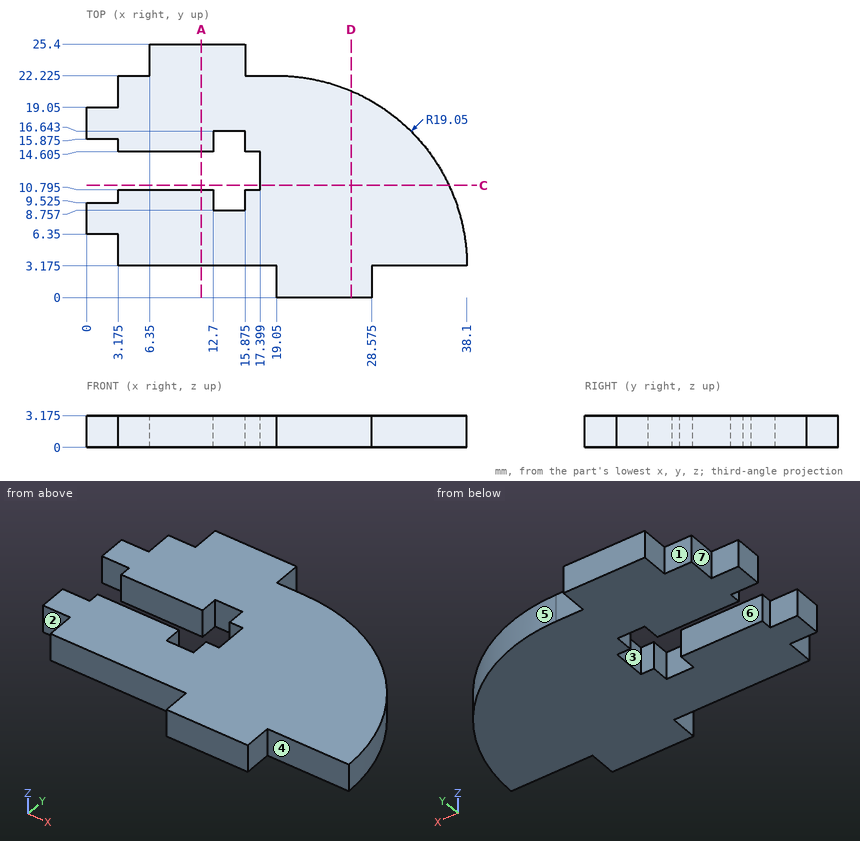
Geometry: see drawing. Coordinates: mm, zero at the bounding-box minimum. A direction names the side the tool comes from. Coordinates: 2 decimals unless noted, no trailing zeros. Loops run counter-clockwise (first coordinate to the right, second up) from the corner with the lowest first, then second, coordinate; pieces in that order, holes last. Notation, with made-up numbers: M 66.5,21.25 L 86.5,21.25 A13 cw 86.5,26.25 Z; hole C 46.5,88.25 d1. An arc over 180 degrees is marked long. Answer in a Markdown table with one row per item.
Q1. Section A-A on x = 11.5. Return the cut outline in (y, z) (1 decimal).
Answers below:
| item | result |
|---|---|
| outline | M 3.2,0 L 10.8,0 L 10.8,3.2 L 3.2,3.2 Z; M 14.6,0 L 25.4,0 L 25.4,3.2 L 14.6,3.2 Z |
Q2. Set-up query: the marked faces 1, 2, 3 and 4. Return all of +Z, -Z, +X, -X, +Y, -Y with unobstructed straight access to the full face (end or side cutting, diameter ignored); none if empty.
Answers below:
| item | result |
|---|---|
| face 1 | +Z, -Z, -X, +Y |
| face 2 | +Z, -Z, -X, -Y |
| face 3 | +Z, -Z, -X |
| face 4 | +Z, -Z, +X, -Y |
Q3. Section C-C on y = 11.25. Return the cut outline in (x, z) (1 decimal).
Answers below:
| item | result |
|---|---|
| outline | M 17.4,0 L 36.3,0 L 36.3,3.2 L 17.4,3.2 Z |
Q4. First-contact query: pin 1 (1 mm diameter, centred on y = 24, z = 2, fed in from -X); pin 2 (1.6 mm diameter, centred on y = 10, z = 1.5, fed in from +X); pin 3 (1 mm diameter, centred on y = 16, z = 2, fed in from +X) (1 decimal). Flat tips, straight axial feed; report the tip coordinate or a pass-through.
Answers below:
| item | result |
|---|---|
| pin 1 | stops at x = 6.35 |
| pin 2 | stops at x = 37.12 |
| pin 3 | stops at x = 33.6 |
Q5. Draft query along Y for the marked faces 5, 6 and 7. Return one class per face: pulls with the +Y half, pulls with the -Y half, needs draft (parallel to the pull), parting line crosses it, or undercut.
Answers below:
| item | result |
|---|---|
| face 5 | pulls with the +Y half |
| face 6 | undercut |
| face 7 | needs draft |
Q6. Ray query, probe 1 along Y at (x, z) = (8, 0.65) (1 decimal); probe 2 along X at (y, z) = (9, 1.7) (1 decimal); probe 3 along Y at (x, z) = (19.5, 0.55). Return the intervals inside material, ascending. Write a range as from..to.
Answers below:
| item | result |
|---|---|
| probe 1 | y = 3.2..10.8, 14.6..25.4 |
| probe 2 | x = 0..12.7, 15.9..37.2 |
| probe 3 | y = 0..22.22 |
Q7. Section D-D on x = 26.5. Return the cut outline in (y, z) (1 decimal).
Answers below:
| item | result |
|---|---|
| outline | M 0,0 L 20.7,0 L 20.7,3.2 L 0,3.2 Z |
